```python
from build123d import *

# Parameters (mm, degrees)
F0_W     = 50
F0_H     = 5
F1_DEPTH = 3
F2_W     = 3
F2_H     = 3
F3_DEPTH = 2


with BuildPart() as f1:
    # F0 (on Front) → F1 (new body)
    with BuildSketch(Plane.XZ):
        Rectangle(F0_W, F0_H)
    extrude(amount=F1_DEPTH)

    # F2 (on face) → F3 (join)
    with BuildSketch(Plane.XZ.offset(3)):
        with Locations((-22.5, 0)):
            Rectangle(F2_W, F2_H)
        with Locations((-17.5, 0)):
            Rectangle(F2_W, F2_H)
        with Locations((-12.5, 0)):
            Rectangle(F2_W, F2_H)
        with Locations((-7.5, 0)):
            Rectangle(F2_W, F2_H)
        with Locations((-2.5, 0)):
            Rectangle(F2_W, F2_H)
        with Locations((2.5, 0)):
            Rectangle(F2_W, F2_H)
        with Locations((7.5, 0)):
            Rectangle(F2_W, F2_H)
        with Locations((12.5, 0)):
            Rectangle(F2_W, F2_H)
        with Locations((17.5, 0)):
            Rectangle(F2_W, F2_H)
        with Locations((22.5, 0)):
            Rectangle(F2_W, F2_H)
    extrude(amount=F3_DEPTH)


solid = f1.part
```
The model under review builds one solid part; all positions refer to its coordinate system, in mm. A direction names the side the tool comes from. Round coordinates to 2 decimals unless told otherwise and drop trailing zeros. Order: outer loops, then holes, each group sorted by start corner. A loop starts at its lowest first (then second) coordinate and runs counter-clockwise, first axis right, second up.
(1) Wall thickness on L1, parallel to Y at x = -15.5, z = 1.6; L2, parallel to Z at x = 7.5, y = -4.6: over which ranges is each line inside the solid? List them lowest first.
Working result:
L1: y = -3 to 0
L2: z = -1.5 to 1.5
(2) For P1, Ø0.6, axis at y = -4, z = -0.5, coming from the -X side; P2, Ø0.6, axis at y = -4, z = 0, coming from the +X side; P3, Ø0.6, axis at x = 7, y = -3.5, coming from the -Z side, all flat-tipped, find the tip position at first contact; note any pin that passes through.
Working result:
P1: stops at x = -24
P2: stops at x = 24
P3: stops at z = -1.5
(3) Take a section at B-B, the plane y = -4. Count the separate pieces of the cut face and the enclosed holes in it, plus the area to 3 significant figures.
Working result:
separate pieces: 10
enclosed holes: 0
area: 90.0 mm2
(4) Take a section at C-C, the plane z = -2. State the section outline as (x, y) points.
Working result:
outline: (-25, -3) - (25, -3) - (25, 0) - (-25, 0) - close
(5) Take a section at A-A, the plane x = -22. State the section outline as (y, z) points.
Working result:
outline: (-5, -1.5) - (-3, -1.5) - (-3, -2.5) - (0, -2.5) - (0, 2.5) - (-3, 2.5) - (-3, 1.5) - (-5, 1.5) - close
(6) Take a section at D-D, the plane x = -10.5. State the section outline as (y, z) points, plus the area to 3 significant figures.
Working result:
outline: (-3, -2.5) - (0, -2.5) - (0, 2.5) - (-3, 2.5) - close
area: 15.0 mm2
(7) Tool access review of faces 4 (the face through (24, -4, 0)), 5 (the face through (2, -4, 1.5)), 6 (the face through (-24, -4, 0)), 7 (the face through (4, -4, 0)), 8 (the face through (-8, -4, -1.5)): name each direction out of +Z, -Z, +X, -X, +Y, -Y from which nothing blocks a thin tool from reaching the whole face with its end or side.
Working result:
face 4: +Z, -Z, +X, -Y
face 5: +Z, +X, -X, -Y
face 6: +Z, -Z, -X, -Y
face 7: +Z, -Z, -Y
face 8: -Z, +X, -X, -Y
(8) Mouldability with a two-part tool opening along X and no side actions: class faces 1 (the face through (-25, -1, 0)), 2 (the face through (-13, -5, 0)), 3 (the face through (-14, -4, 0)) as released by +X, released by -X, zero draft, split by the parting line, or undercut.
Working result:
face 1: released by -X
face 2: zero draft
face 3: undercut
